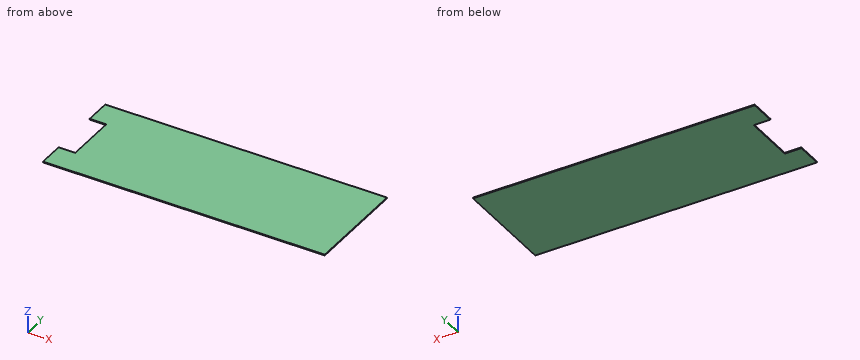
Autodesk Inventor part; units mm, degrees
ref_plane "YZ Plane" through (0, 0, 0) normal (1, 0, 0) x (0, 1, 0)
ref_plane "XZ Plane" through (0, 0, 0) normal (0, 1, 0) x (-1, 0, 0)
ref_plane "XY Plane" through (0, 0, 0) normal (0, 0, 1) x (1, 0, 0)
sketch "Sketch1" plane through (0, 0, 0) normal (0, 0, 1) x (1, 0, 0)
  line L0 (-116.7504, -3.6908) -> (-895.8037, -3.6908)
  line L1 (-895.8037, -3.6908) -> (-895.8037, 301.1092)
  line L2 (-895.8037, 301.1092) -> (-116.7504, 301.1092)
  line L3 (-116.7504, 301.1092) -> (-116.7504, -3.6908)
  line L4 (-895.8037, -3.6908) -> (-944.7633, -3.6908)
  line L5 (-944.7633, -3.6908) -> (-944.7633, 72.5092)
  line L6 (-944.7633, 72.5092) -> (-895.8037, 72.5092)
  line L7 (-895.8037, 72.5092) -> (-895.8037, -3.6908)
  line L8 (-895.8037, 301.1092) -> (-944.7633, 301.1092)
  line L9 (-944.7633, 301.1092) -> (-944.7633, 224.9092)
  line L10 (-944.7633, 224.9092) -> (-895.8037, 224.9092)
  line L11 (-895.8037, 224.9092) -> (-895.8037, 301.1092)
  line L12 (-116.5344, 301.1092) -> (-116.5344, -3.6908)
  point P0 (0, 0)
  dimension "d1" = 304.8
  dimension "d4" = 76.2
  dimension "d5" = 76.2
extrude "Extrusion1" add sketch "Sketch1" along normal blind 2.54
properties part number "plexiglass2" material "Glass"
Verification items for the finished model (mm, model axes). Coordinates: 2 decimals unless noted, no trailing zeros. Write each loop counter-clockwise with the first axis right and the second up, starting at its lowest first coordinate (ties: lowest second). Pieces come first, ordered by that corner, then holes. Notation, with made-up numbers: (19.5, 3) - (31.5, 3) arc R24 ccw to (31.5, 34) - close; hole circle Ø6 at (65, 3). An arc over 180 degrees is marked (long way). Answer as a JSON object with one key per item and string values.
(1) Cross-section at A-A on z = 1.45. Record the cut outline in (x, y).
Report:
{"outline": "(-944.76, -3.69) - (-116.75, -3.69) - (-116.75, 301.11) - (-944.76, 301.11) - (-944.76, 224.91) - (-895.8, 224.91) - (-895.8, 72.51) - (-944.76, 72.51) - close"}
(2) Thickness scan on line 1 along X through (y, z) = (205.5, 0.8); line 2 along Y through (x, z) = (-911, 0.35). Record the ranges inside material, lowest first.
Report:
{"line 1": "-895.8 to -116.75", "line 2": "-3.69 to 72.51, 224.91 to 301.11"}
(3) Cross-section at B-B on y = 115. Record the cut outline in (x, z), plus the area to 3 significant figures.
Report:
{"outline": "(-895.8, 0) - (-116.75, 0) - (-116.75, 2.54) - (-895.8, 2.54) - close", "area": "1,980 mm^2"}
(4) Gauge pin test, flat ends, axial feed: pin 1 Ø1.5 at (y, z) = (148, 1.5) entering from -X; pin 2 Ø5 at (x, y) = (-642.5, 74.5) entering from -Z. Record the tip position at first contact, or that the pin passes through.
Report:
{"pin 1": "x = -895.8", "pin 2": "z = 0"}
